```python
from build123d import *

# Parameters (mm, degrees)
F0_R      = 11.5
F0_R_2    = 2.1
F1_DEPTH  = 7
F2_R      = 10.5
F3_DEPTH  = 5
F5_DEPTH  = 7
F6_W      = 8.5
F6_H      = 2
F7_DEPTH  = 12.8
F8_W      = 6.5
F8_H      = 5
F9_DEPTH  = 15
F10_W     = 1
F10_H     = 5
F11_DEPTH = 0.5
F12_W     = 1
F12_H     = 5
F13_DEPTH = 0.5
F14_SIZE  = 0.49999
F15_SIZE  = 1


# Not quite as in the source:
# - a fillet or chamfer is up to 0.001 mm smaller than in the source, because OpenCascade refuses the exact size


with BuildPart() as f1:
    # F0 (on Top) → F1 (new body)
    with BuildSketch(Plane.XY):
        Circle(F0_R)
        Circle(F0_R_2, mode=Mode.SUBTRACT)
    extrude(amount=F1_DEPTH)

    # F2 (on face) → F3 (cut)
    with BuildSketch(Plane.XY.offset(7)):
        Circle(F2_R)
    extrude(amount=-F3_DEPTH, mode=Mode.SUBTRACT)

    # F4 (on face) → F5 (join)
    with BuildSketch(Plane.XY.offset(7)):
        with BuildLine():
            Line((-11.5, 16), (-11.5, 0))
            ThreePointArc((-11.5, 0), (-11.2472218792, 2.3979157617), (-10.5, 4.6904157598))
            Line((-10.5, 4.6904157598), (-10.5, 16))
            Line((-10.5, 16), (-11.5, 16))
        make_face()
        with BuildLine():
            ThreePointArc((-4, 10.7819293264), (-3.5036523196, 10.9532835453), (-3, 11.1018016556))
            Line((-3, 11.1018016556), (-3, 16))
            Line((-3, 16), (-4, 16))
            Line((-4, 16), (-4, 10.7819293264))
        make_face()
    extrude(amount=-F5_DEPTH)

    # F6 (on face) → F7 (join)
    with BuildSketch(Plane(origin=(0, 16, 0), x_dir=(-1, 0, 0), z_dir=(0, 1, 0))):
        with Locations((7.25, 1)):
            Rectangle(F6_W, F6_H)
    extrude(amount=-F7_DEPTH)

    # F8 (on face) → F9 (cut)
    with BuildSketch(Plane(origin=(0, 16, 0), x_dir=(-1, 0, 0), z_dir=(0, 1, 0))):
        with Locations((7.25, 4.5)):
            Rectangle(F8_W, F8_H)
    extrude(amount=-F9_DEPTH, mode=Mode.SUBTRACT)

    # F10 (on face) → F11 (join)
    with BuildSketch(Plane.YZ.offset(-10.5)):
        with Locations((1.5, 4.5)):
            Rectangle(F10_W, F10_H)
        with Locations((15.5, 4.5)):
            Rectangle(F10_W, F10_H)
    extrude(amount=F11_DEPTH)

    # F12 (on face) → F13 (join)
    with BuildSketch(Plane(origin=(-4, 0, 0), x_dir=(0, -1, 0), z_dir=(-1, 0, 0))):
        with Locations((-15.5, 4.5)):
            Rectangle(F12_W, F12_H)
    extrude(amount=F13_DEPTH)

    # F14 (size 0.5 in the source; OpenCascade refuses exactly that, so slightly less here)
    f14_edges = [f1.edges().sort_by_distance(p)[0] for p in [
        (-10, 1.5, 7),
        (-10, 15.5, 7),
        (-4.5, 15.5, 7),
    ]]
    chamfer(f14_edges, length=F14_SIZE)

    # F15
    f15_edges = [f1.edges().sort_by_distance(p)[0] for p in [
        (9.130991, -6.991066, 0),
        (-3, 13.550901, 0),
        (-11.5, 8, 0),
    ]]
    chamfer(f15_edges, length=F15_SIZE)


solid = f1.part
```
Can you work these out from the model? Positions are in its coordinate system, mm. A direction names the side the tool comes from. Coordinates: 2 decimals unless noted, no trailing zeros. Loops run counter-clockwise (first coordinate to the right, second up) from the corner with the lowest first, then second, coordinate; pieces in that order, holes last. Notation, with made-up numbers: (27, 32.5) - (71, 32.5) arc R36 ccw to (71, 70.5) - close; hole circle Ø6 at (86.25, 27.5). An arc over 180 degrees is marked (long way). Use a Markdown table: item, result.
Item 1: For faces 4 (the face through (-10, 15.5, 4.3)), 5 (the face through (8.204, -6.554, 4.535)), 6 (the face through (8.65, -6.25, 0.17)), which set-ups out of +Z, -Z, +X, -X, +Y, -Y let a thin tool reach every point of the face, with its end or its side?
Numbers:
| item | result |
|---|---|
| face 4 | +Z, +Y |
| face 5 | +Z |
| face 6 | -Z |
Item 2: I want a section at A-A on x = 0. Please give me the cut outline in (y, z).
Numbers:
| item | result |
|---|---|
| outline | (-11.5, 1) - (-10.5, 0) - (-2.1, 0) - (-2.1, 2) - (-10.5, 2) - (-10.5, 7) - (-11.5, 7) - close; (2.1, 0) - (10.5, 0) - (11.5, 1) - (11.5, 7) - (10.5, 7) - (10.5, 2) - (2.1, 2) - close |
Item 3: We'd pull the mould along Y, two halves only. Please class faces 1 (the face through (0, 3, 0)), 2 (the face through (-7, 16, 1)), 3 (the face through (-10.5, 8, 5)): released by +Y, released by -Y, zero draft, split by the parting line, or undercut.
Numbers:
| item | result |
|---|---|
| face 1 | zero draft |
| face 2 | released by +Y |
| face 3 | undercut |
Item 4: If I drill on probe 1 along Y at (x, z) = (0, 4.5); probe 2 along Y at (x, z) = (0, 1.3), over which ranges is the centre line in solid material (lowest first)? Write a range as from..to.
Numbers:
| item | result |
|---|---|
| probe 1 | y = -11.5..-10.5, 10.5..11.5 |
| probe 2 | y = -11.5..-2.1, 2.1..11.5 |
Item 5: Will these pins go through, and if not, where does the flat tip stop? pin 1 (0.8 mm diameter, centred on y = 1.5, z = 5, fed in from +X); pin 2 (4 mm diameter, centred on y = 10, z = 5, fed in from +X); pin 3 (10.5 mm diameter, centred on x = 0.5, y = -3.5, fed in from +Z); pin 4 (1.5 mm diameter, centred on x = 1.5, y = 13, fed in from -Z).
Numbers:
| item | result |
|---|---|
| pin 1 | stops at x = 11.45 |
| pin 2 | stops at x = 8.26 |
| pin 3 | stops at z = 2 |
| pin 4 | passes through |
Item 6: I want a section at B-B on z = 4.75. Please give me the cut outline in (x, y).
Numbers:
| item | result |
|---|---|
| outline | (-11.5, 0) arc R11.5 ccw (long way) to (-3, 11.1) - (-3, 16) - (-4.5, 16) - (-4.5, 15) - (-4, 15) - (-4, 9.71) arc R10.5 cw (long way) to (-10.45, 1) - (-10, 1) - (-10, 2) - (-10.5, 2) - (-10.5, 15) - (-10, 15) - (-10, 16) - (-11.5, 16) - close |
